Autodesk Inventor part; units mm, degrees
ref_plane "YZ Plane" through (0, 0, 0) normal (1, 0, 0) x (0, 1, 0)
ref_plane "XZ Plane" through (0, 0, 0) normal (0, 1, 0) x (-1, 0, 0)
ref_plane "XY Plane" through (0, 0, 0) normal (0, 0, 1) x (1, 0, 0)
sketch "Sketch2" plane through (0, 0, 0) normal (0, 1, 0) x (-1, 0, 0)
  line L0 (0, 0) -> (0, -812.8)
  line L1 (19.05, 19.05) -> (19.05, -831.85)
  line L2 (19.05, -831.85) -> (0, -812.8)
  line L3 (19.05, 19.05) -> (0, 0)
  point P0 (19.05, -406.4)
  point P1 (0, -406.4)
  dimension "d2" = 812.8
  dimension "d3" = 850.9
  dimension "d4" = 19.05
extrude "Extrusion1" add sketch "Sketch2" along normal blind 127
sketch "Sketch3" plane through (0, 0, 0) normal (1, 0, 0) x (0, 0, -1)
  line L0 (0, 0) -> (812.8, 0) construction
  line L1 (812.8, 0) -> (812.8, 127) construction
  line L2 (0, 127) -> (812.8, 127) construction
  line L3 (0, 0) -> (0, 127) construction
  line L4 (0, 77.2583) -> (12.7, 77.2583) construction
  circle A0 centre (12.7, 77.2583) radius 1.905
  circle A1 centre (57.15, 77.2583) radius 1.905
  circle A2 centre (101.6, 77.2583) radius 1.905 construction
  circle A3 centre (12.7, 49.7417) radius 1.905
  circle A4 centre (57.15, 49.7417) radius 1.905
  circle A5 centre (101.6, 49.7417) radius 1.905 construction
  line L5 (406.4, 127) -> (406.4, 0) construction
  circle A6 centre (800.1, 77.2583) radius 1.905
  circle A7 centre (755.65, 77.2583) radius 1.905
  circle A8 centre (711.2, 77.2583) radius 1.905 construction
  circle A9 centre (800.1, 49.7417) radius 1.905
  circle A10 centre (755.65, 49.7417) radius 1.905
  circle A11 centre (711.2, 49.7417) radius 1.905 construction
  line L6 (12.7, 77.2583) -> (12.7, 49.7417) construction
  line L7 (-19.05, 0) -> (-19.05, 127)
  point P0 (12.7, 63.5)
  dimension "d9" = 3.81
  dimension "d12" = 44.45
  dimension "d15" = 27.5167
  dimension "d23" = 63.5
  dimension "d24" = 31.75
extrude "Extrusion2" cut sketch "Sketch3" against normal blind 127
sketch "Sketch4" plane through (0, 127, 0) normal (0, 1, 0) x (1, 0, 0)
  line L0 (-19.05, 831.85) -> (-19.05, -19.05)
  line L1 (-19.05, 406.4) -> (0, 406.4)
  line L2 (0, 0) -> (0, 812.8)
  line L3 (0, 0) -> (0, 812.8)
  line L4 (0, 812.8) -> (-19.05, 831.85)
  line L5 (-19.05, 831.85) -> (-19.05, -19.05)
  line L6 (-19.05, -19.05) -> (0, 0)
  line L7 (-19.05, 404.8125) -> (0, 404.8125)
  point P0 (-19.05, 404.8125)
  point P1 (0, 404.8125)
  dimension "d22" = 1.5875
extrude "Extrusion3" cut sketch "Sketch4" against normal blind 127 contours L4 L2 L1 L0 | L1 L2 L7 L0
properties part number "BUMP_002_Wood2" material "Wood (Birch)"
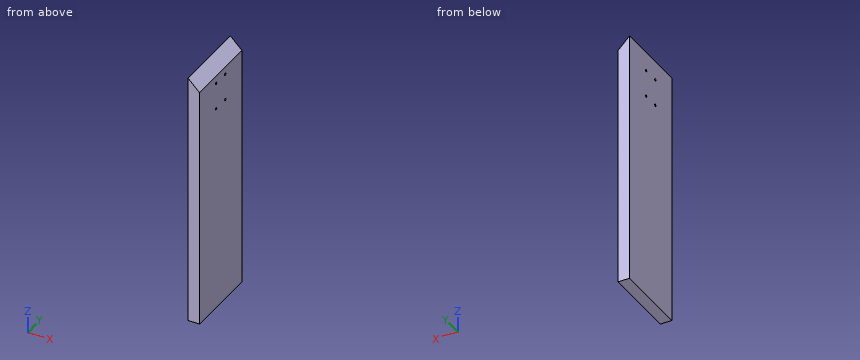
Geometry: final body of the model. Coordinates: model frame, mm. Round coordinates to 2 decimals unless told otherwise and drop trailing zeros. Order: outer loops, then holes, each group sorted by start corner. A loop starts at its lowest first (then second) coordinate and runs counter-clockwise, first axis right, second up. Notation, with made-up numbers: (34.5, -7) -> (89.5, -7) arc R37 cw to (89.5, 32) -> close; hole circle Ø10 at (64, 53.25). An arc over 180 degrees is marked (long way). Use one line per item in the form item = value. Start each with the question number.
1. Cut plane A-A (x = -11.75). Count the separate pieces of the cut face and the enclosed holes in it, then the cut area to 3 significant figures.
2. Cut plane B-B (y = 102). Return the cut outline in (x, z).
3. Line query: probe 1 along Y at (x, z) = (-3.75, -57.15); probe 2 along Z at (x, y) = (-14, 106.5); probe 3 along Z at (x, y) = (-15.25, 80.5). Output: solid intervals per line, ascending.
4. Pin query (flat end, axial travel): pin 1 Ø4 at (x, y) = (-6.5, 98.5) entering from +Z; pin 2 Ø4 at (x, z) = (-4.5, -197) entering from -Y. Return the tip coordinate at first contact, or that it passes through.
Solution:
q1.separate_pieces = 1
q1.enclosed_holes = 4
q1.area = 52,900 mm^2
q2.outline = (-19.05, -404.81) -> (0, -404.81) -> (0, 0) -> (-19.05, 19.05) -> close
q3.probe_1 = 0 to 47.84, 51.65 to 75.35, 79.16 to 127
q3.probe_2 = -404.81 to 14
q3.probe_3 = -404.81 to 15.25
q4.pin_1 = 8.5
q4.pin_2 = 0
